```python
from build123d import *

# Parameters (mm, degrees)
F0_R          = 20
F1_DEPTH      = 40
F3_DEPTH      = 30
F4_R          = 10
F5_DEPTH      = 40.001
F6_W          = 20
F6_H          = 10
F7_DEPTH      = 20.001
F7_DEPTH_BACK = 40.001


with BuildPart() as f1:
    # F0 (on Front) → F1 (new body)
    with BuildSketch(Plane.XZ):
        Circle(F0_R)
    extrude(amount=F1_DEPTH)

    # F2 (on face) → F3 (join)
    with BuildSketch(Plane(origin=(0, 0, 0), x_dir=(-1, 0, 0), z_dir=(0, 1, 0))):
        with BuildLine():
            ThreePointArc((0, -20), (-20, 0), (0, 20))
            Line((0, 20), (-30, 20))
            Line((-30, 20), (-40, 10))
            Line((-40, 10), (-40, -10))
            Line((-40, -10), (-30, -20))
            Line((-30, -20), (0, -20))
        make_face()
    extrude(amount=-F3_DEPTH)

    # F4 (on face) → F5 (cut, through all)
    with BuildSketch(Plane.XZ.offset(40)):
        Circle(F4_R)
    extrude(amount=-F5_DEPTH, mode=Mode.SUBTRACT)

    # F6 (on Right) → F7 (cut, two sides)
    with BuildSketch(Plane.YZ) as f7_sk:
        with Locations((-30, 0)):
            Rectangle(F6_W, F6_H)
    extrude(amount=-F7_DEPTH, mode=Mode.SUBTRACT)
    extrude(f7_sk.sketch, amount=F7_DEPTH_BACK, mode=Mode.SUBTRACT)


solid = f1.part
```
Design review of the part built by this model. Coordinates are the model's own, in mm. A direction names the side the tool comes from. Round coordinates to 2 decimals unless told otherwise and drop trailing zeros. Write each loop counter-clockwise with the first axis right and the second up, starting at its lowest first coordinate (ties: lowest second). Pieces come first, ordered by that corner, then holes.
Item 1: For probe 1 along X at (y, z) = (-11.5, 0); probe 2 along Z at (x, y) = (-5, -31); probe 3 along Y at (x, z) = (23, -12), list the stretches that pass through material, from the lowest coordinate up.
Item 2: For faces 4 (the cylindrical face through (-19.984, -19.72, 0.809)), 5 (the flat face through (15, -15, 20)), 6 (the flat face through (25, -30, -12)), 7 (the flat face through (25, -30, 13)), 8 (the flat face through (21, -28, -5)), list the 3-axis set-ups (+Z, -Z, +X, -X, +Y, -Y) from which the entire face can be reached by the end or side of a thin tool; tool diameter is ignored.
Item 3: We need section C-C on x = 3. Write out the cut boundary in (y, z).
Item 4: We need section D-D on y = -21. Write out the cut boundary in (x, z), and give its area (3 significant figures).
Item 5: We need section A-A on y = -31. Write out the cut boundary in (x, z), and give its area (3 significant figures).
Item 6: The part is to be moulded in two halves that separate along Z. For faces 1 (the flat face through (35, -15, -15)), 2 (the flat face through (40, -11, 0)), 3 (the flat face through (-14, -30, -5)), say which applies: +Z half, -Z half, draft (parallel to the pull), parting line (faces both ways), or undercut.
Item 7: We need section B-B on z = 0. Write out the cut boundary in (x, y), and give its area (3 significant figures).
Item 8: Clearance check with flat-ended pins moving along their axes: pin 1 Ø8 at (y, z) = (-5, 6) entering from -X; pin 2 Ø8 at (x, z) = (-13, 0.5) entering from -Y; pin 3 Ø12 at (x, y) = (-14.5, -29.5) entering from +Z; pin 4 Ø3 at (y, z) = (-22.5, 1.5) entering from +X. State where each tip first meets the part, or that it passes through.
Returned:
1. probe 1: x = -20 to -10, 10 to 40
1. probe 2: z = -19.36 to -8.66, 8.66 to 19.36
1. probe 3: y = -30 to 0
2. face 4: -Y
2. face 5: +Z, +X, -X, +Y, -Y
2. face 6: -Z, +X, -Y
2. face 7: +Z, +X, -Y
2. face 8: +X, -X, -Y
3. outline: (-40, -19.77) - (-30, -19.77) - (-30, -20) - (0, -20) - (0, -9.54) - (-40, -9.54) - close; (-40, 9.54) - (0, 9.54) - (0, 20) - (-30, 20) - (-30, 19.77) - (-40, 19.77) - close
4. outline: (-19.36, -5) arc R20 ccw to (0, -20) - (30, -20) - (40, -10) - (40, -5) - (8.66, -5) arc R10 cw to (-8.66, -5) - close; (-19.36, 5) - (-8.66, 5) arc R10 cw to (8.66, 5) - (40, 5) - (40, 10) - (30, 20) - (0, 20) arc R20 ccw to start
4. area: 1,410 mm2
5. outline: (-19.36, -5) arc R20 ccw to (19.36, -5) - (8.66, -5) arc R10 cw to (-8.66, -5) - close; (-19.36, 5) - (-8.66, 5) arc R10 cw to (8.66, 5) - (19.36, 5) arc R20 ccw to start
5. area: 738 mm2
6. face 1: -Z half
6. face 2: draft
6. face 3: undercut
7. outline: (-20, -20) - (-10, -20) - (-10, 0) - (-20, 0) - close; (10, -20) - (40, -20) - (40, 0) - (10, 0) - close
7. area: 800 mm2
8. pin 1: stops at x = -19.9
8. pin 2: stops at y = -20
8. pin 3: stops at z = 18.1
8. pin 4: passes through
